Here's how the part is built. I have some questions about the finished solid (model axes, mm). A direction names the side the tool comes from. Round coordinates to 2 decimals unless told otherwise and drop trailing zeros. Write each loop counter-clockwise with the first axis right and the second up, starting at its lowest first coordinate (ties: lowest second). Pieces come first, ordered by that corner, then holes. Notation, with made-up numbers: (3.5, -1) -> (37.5, -1) arc R19 cw to (37.5, 21) -> close; hole circle Ø4 at (40, -16). An arc over 180 degrees is marked (long way). Answer as CSV lines item,"result".
Autodesk Fusion 360 part; units mm, degrees
sketch "Sketch1" plane through (0, 0, 0) normal (0, 0, 1) x (1, 0, 0)
  line L0 (-13.1, 18.85) -> (-11.1, 18.85)
  line L1 (-11.1, 18.85) -> (-11.1, -18.85)
  line L2 (-11.1, -18.85) -> (-13.1, -18.85)
  line L3 (-13.1, -18.85) -> (-13.1, 18.85)
  line L4 (-13.1, -18.85) -> (13.1, -18.85)
  line L5 (13.1, -18.85) -> (13.1, -16.85)
  line L6 (13.1, -16.85) -> (-13.1, -16.85)
  line L7 (-13.1, -16.85) -> (-13.1, -18.85)
  line L8 (13.1, -18.85) -> (11.1, -18.85)
  line L9 (11.1, -18.85) -> (11.1, 35.15)
  line L10 (11.1, 35.15) -> (13.1, 35.15)
  line L11 (13.1, 35.15) -> (13.1, -18.85)
  line L12 (13.1, 35.15) -> (-11.2, 35.15)
  line L13 (-11.2, 35.15) -> (-11.2, 33.15)
  line L14 (-11.2, 33.15) -> (13.1, 33.15)
  line L15 (13.1, 33.15) -> (13.1, 35.15)
  line L16 (-11.1, 16.65) -> (11.1, 16.65)
  line L17 (11.1, 16.65) -> (11.1, 14.65)
  line L18 (11.1, 14.65) -> (-11.1, 14.65)
  line L19 (-11.1, 14.65) -> (-11.1, 16.65)
  dimension "d1" = 2
  dimension "d2" = 2
  dimension "d3" = 2
  dimension "d4" = 2
  dimension "d5" = 2
  dimension "d6" = 26.2
  dimension "d7" = 37.7
  dimension "d8" = 35.5
  dimension "d9" = 54
  dimension "d10" = 24.3
  dimension "d36" = 13.1
  dimension "d37" = 18.85
extrude "Extrude1" add sketch "Sketch1" along normal mid plane 20 contours L0 L1 L3 L6 L19 | L1 L2 L3 L4 L6 L7 | L1 L9 L16 L17 L18 L19 | L1 L4 L6 L9 | L6 L9 L11 L14 L17 | L4 L5 L6 L8 L9 L11 | L9 L12 L13 L14 | L9 L10 L11 L12 L14 L15
sketch "Sketch2" plane through (0, 14.65, 0) normal (0, -1, 0) x (1, 0, 0)
  line L0 (-11.1, -10) -> (11.1, -10)
  line L1 (11.1, -10) -> (11.1, 10)
  line L2 (11.1, 10) -> (-11.1, 10)
  line L3 (-11.1, 10) -> (-11.1, -10)
  circle A0 centre (0, 0) radius 10
  dimension "d13" = 20
  dimension "d14" = 10
  dimension "d15" = 22.2
  dimension "d16" = 11.1
extrude "Extrude2" add sketch "Sketch2" along normal blind 32 contours A0
fillet "Fillet1" radius 1.5 3 edges at (-13.1, -18.85, 0) (13.1, -18.85, 0) (13.1, 35.15, 0)
sketch "Sketch3" plane through (0, 16.65, 0) normal (0, 1, 0) x (-1, 0, 0)
  line L0 (-11.1, -10) -> (11.1, -10)
  line L1 (11.1, -10) -> (11.1, 10)
  line L2 (11.1, 10) -> (-11.1, 10)
  line L3 (-11.1, 10) -> (-11.1, -10)
  line L4 (-11.6, -10) -> (-13.1, -10)
  line L5 (-11.6, -10) -> (11.6, -10)
  line L6 (13.1, -10) -> (11.6, -10)
  line L7 (-13.1, -10) -> (-13.1, 10)
  line L8 (-13.1, 10) -> (-11.6, 10)
  line L9 (11.6, 10) -> (13.1, 10)
  line L10 (13.1, 10) -> (13.1, -10)
  line L11 (11.6, 10) -> (-11.6, 10)
  circle A0 centre (0, 0) radius 4
  arc A1 (0, -10) -> (0, 10) centre (0, 0) ccw
  arc A2 (0, 10) -> (0, -10) centre (0, 0) ccw
  arc A3 (0, -10) -> (0, 10) centre (0, 0) ccw
  arc A4 (0, 10) -> (0, -10) centre (0, 0) ccw
  dimension "d20" = 8
extrude "Extrude3" add sketch "Sketch3" along normal blind 15 contours A0
sketch "Sketch5" plane through (0, 35.15, 0) normal (0, 1, 0) x (-1, 0, 0)
  line L0 (-11.6, 10) -> (-11.6, -10)
  line L1 (-11.6, -10) -> (11.2, -10)
  line L2 (11.2, -10) -> (11.2, 10)
  line L3 (11.2, 10) -> (-11.6, 10)
  circle A0 centre (0, 0) radius 4
  circle A1 centre (0, 0) radius 4
  line L4 (5.15, 5.15) -> (-5.15, 5.15)
  line L5 (-5.15, 5.15) -> (-5.15, -5.15)
  line L6 (-5.15, -5.15) -> (5.15, -5.15)
  line L7 (5.15, -5.15) -> (5.15, 5.15)
  line L8 (5.15, 5.15) -> (-5.15, -5.15) construction
  line L9 (-5.15, 5.15) -> (5.15, -5.15) construction
  dimension "d30" = 10.3
  dimension "d31" = 10.3
extrude "Extrude5" cut sketch "Sketch5" against normal blind 4 contours A0 A1 | L4 L5 L6 L7
sketch "Sketch4" plane through (0, 0, 0) normal (0, 0, 1) x (1, 0, 0)
  line L0 (-5, 30.65) -> (5, 30.65)
  line L1 (5, 30.65) -> (5, 44.65)
  line L2 (5, 44.65) -> (-5, 44.65)
  line L3 (-5, 44.65) -> (-5, 30.65)
  line L4 (5, 44.65) -> (-5, 38.65)
  line L5 (-11.1, 16.65) -> (11.1, 16.65)
  dimension "d23" = 10
  dimension "d26" = 14
  dimension "d27" = 8
  dimension "d35" = 28
  dimension "d38" = 5
extrude "Extrude4" add sketch "Sketch4" along normal mid plane 10 contours L0 L1 L3 L4
sketch "Sketch6" plane through (13.1, 0, 0) normal (1, 0, 0) x (0, 1, 0)
  line L0 (33.65, -10) -> (33.65, 10)
  line L1 (33.65, 10) -> (-17.35, 10)
  line L2 (-17.35, 10) -> (-17.35, -10)
  line L3 (-17.35, -10) -> (33.65, -10)
  line L4 (35.15, -10) -> (35.15, 10)
  point P0 (-8.35, 6.5)
  point P1 (11.65, 6.5)
  point P2 (11.65, -6.5)
  point P3 (-8.35, -6.5)
  dimension "d39" = 13
  dimension "d40" = 6.5
  dimension "d41" = 20
  dimension "d42" = 23.5
  dimension "d46" = 13
hole "Hole1" at (13.1, 11.65, 6.5) at (13.1, 11.65, -6.5) at (13.1, -8.35, -6.5) at (13.1, -8.35, 6.5) direction (-1, 0, 0) diameter 2.529 depth 2 tip angle 180
equation "d2 = d1"
equation "d3 = d1"
equation "d4 = d1"
equation "d5 = d1"
equation "d36 = d6 / 2"
equation "d37 = d7 / 2"
equation "d38 = d23 / 2"
equation "d40 = d39 / 2"
equation "d46 = d39"
Item 1: I need wall thicknesses on L1, parallel to Z at x = 11.5, y = 11.65; L2, parallel to Y at x = 11.75, z = -6.5; L3, parallel to Y at x = 9, z = -6. Which ranges of each line are inside material? Lowest first, please.
Results found:
L1,"z = -10 to -7.76, -5.24 to 5.24, 7.76 to 10"
L2,"y = -18.84 to -9.61, -7.09 to 10.39, 12.91 to 35.14"
L3,"y = -18.85 to -16.85, 14.65 to 16.65, 33.15 to 35.15"
Item 2: Will these pins go through, and if not, where does the flat tip stop? pin 1 (12 mm diameter, centred on x = -4, y = -9, fed in from +Z); pin 2 (3.5 mm diameter, centred on x = -3.5, z = -1, fed in from +Y); pin 3 (5 mm diameter, centred on x = -3.5, z = -5.5, fed in from +Y); pin 4 (11 mm diameter, centred on x = 0.5, y = 41, fed in from -Z).
Results found:
pin 1,"stops at z = 10"
pin 2,"stops at y = 40.6"
pin 3,"stops at y = 41.02"
pin 4,"stops at z = -5"
Item 3: If we mould it in two halves opening along Y, with no side actions, what happens to faces 6 (the cylindrical face through (12.086, -7.116, 6.774)), 7 (the flat face through (0, 36, -5)), 8 (the flat face through (0.07, 41.69, -0.07)), 9 (the cylindrical face through (-12.67, -18.4, 0.14))? For each: pulls with the +Y half, pulls with the -Y half, needs draft (parallel to the pull), parting line crosses it, or undercut.
Results found:
face 6,"undercut"
face 7,"needs draft"
face 8,"pulls with the +Y half"
face 9,"pulls with the -Y half"
Item 4: Suppose I cut it at A-A, the plane z = 0. State how many separate pieces and enclosed holes the cut face has, then the cut area to 3 significant figures.
Results found:
separate pieces,"2"
enclosed holes,"2"
area,"1,150 mm²"
Item 5: Suppose I cut it at B-B, the plane y = 26. List the corners of the cut face in (x, z) for me, then the cut area to 3 significant figures.
Results found:
outline,"circle Ø8 at (0, 0); (11.1, -10) -> (13.1, -10) -> (13.1, 10) -> (11.1, 10) -> close"
area,"90.3 mm²"
Item 6: Suppose I cut it at D-D, the plane y = 6.5. List the corners of the cut face in (x, z) for me, then the cut area to 3 significant figures.
Results found:
outline,"(-13.1, -10) -> (-11.1, -10) -> (-11.1, 10) -> (-13.1, 10) -> close; circle Ø20 at (0, 0); (11.1, -10) -> (13.1, -10) -> (13.1, 10) -> (11.1, 10) -> close"
area,"394 mm²"
Item 7: For faces 1 (the cylindrical face through (0.867, 23.552, 3.905)), 2 (the cylindrical face through (12.086, 12.419, 7.503)), 3 (the flat face through (0, 34, -5.15)), 4 (the flat face through (-11.1, -1, 0)), 5 (the flat face through (0, -18.85, 0)), which set-ups out of +Z, -Z, +X, -X, +Y, -Y let a thin tool reach every point of the face, with its end or its side?
Results found:
face 1,"none"
face 2,"+X"
face 3,"+Y"
face 4,"+Z, -Z"
face 5,"+Z, -Z, +X, -X, -Y"
Item 8: Suppose I cut it at C-C, the plane x = -6. List the corners of the cut face in (y, z) for me.
Results found:
outline,"(-18.85, -10) -> (-16.85, -10) -> (-16.85, -8) -> (14.65, -8) -> (14.65, -10) -> (16.65, -10) -> (16.65, 10) -> (14.65, 10) -> (14.65, 8) -> (-16.85, 8) -> (-16.85, 10) -> (-18.85, 10) -> close; (33.15, -10) -> (35.15, -10) -> (35.15, 10) -> (33.15, 10) -> close"
